Geometry: final body of the model. Coordinates: model frame, mm. A direction names the side the tool comes from. Give positions to 0.01 mm unless a question says otherwise; leave off trailing zeros. Loops run counter-clockwise (first coordinate to the right, second up) from the corner with the lowest first, then second, coordinate; pieces in that order, holes last. Notation, with made-up numbers: M -32.75,87 L -23.75,87 A34 cw -23.75,119 Z; hole C 58.5,-23 d1. An arc over 180 degrees is marked long. Put each result on its own line as item: value.
```python
from build123d import *

# Parameters (mm, degrees)
SKETCH1_W                       = 40.64
SKETCH1_H                       = 17.78
BOSS_EXTRUDE1_DEPTH             = 29.972
SKETCH2_W                       = 26.67
SKETCH2_H                       = 29.972
CUT_EXTRUDE1_DEPTH              = 12.7
SKETCH5_R                       = 8.001
CUT_EXTRUDE4_DEPTH              = 41.340446006
SKETCH6_R                       = 1.1303
CUT_EXTRUDE5_DEPTH              = 52.802457789
SKETCH7_W                       = 19.900329636
SKETCH7_H                       = 4.576555205
BOSS_EXTRUDE2_DEPTH             = 5.08
F_5_32_0_15625_DIAMETER_HOLE1_D = 3.96875
F_30_0_1285_DIAMETER_HOLE1_D    = 3.2639
SKETCH14_W                      = 1.1303
SKETCH14_H                      = 29.972
SKETCH16_W                      = 40.64
SKETCH16_H                      = 26.629644064
CUT_EXTRUDE6_DEPTH              = 41.347520619


with BuildPart() as part:
    # Sketch1 → Boss-Extrude1 (new body)
    with BuildSketch(Plane(origin=(0, 0, 0), x_dir=(1, 0, 0), z_dir=(0, 1, 0))):
        with Locations((0, 2.667)):
            Rectangle(SKETCH1_W, SKETCH1_H)
    extrude(amount=BOSS_EXTRUDE1_DEPTH)

    # Sketch2 → Cut-Extrude1 (cut)
    with BuildSketch(Plane.XY.offset(6.223)):
        with Locations((0, 14.986)):
            Rectangle(SKETCH2_W, SKETCH2_H)
    extrude(amount=-CUT_EXTRUDE1_DEPTH, mode=Mode.SUBTRACT)

    # Sketch5 → Cut-Extrude4 (cut, through all)
    with BuildSketch(Plane(origin=(0, 0, -11.557), x_dir=(-1, 0, 0), z_dir=(0, 0, -1))):
        with Locations((0, 15.875)):
            Circle(SKETCH5_R)
    extrude(amount=-CUT_EXTRUDE4_DEPTH, mode=Mode.SUBTRACT)

    # Sketch6 → Cut-Extrude5 (cut, through all)
    with BuildSketch(Plane.ZY.offset(20.32)):
        with Locations((-2.667, 15.24)):
            Circle(SKETCH6_R)
    extrude(amount=-CUT_EXTRUDE5_DEPTH, mode=Mode.SUBTRACT)

    # Sketch7 → Boss-Extrude2 (add)
    with BuildSketch(Plane.XY.offset(-6.477)):
        with Locations((0, 27.693243708)):
            Rectangle(SKETCH7_W, SKETCH7_H)
    extrude(amount=BOSS_EXTRUDE2_DEPTH)

    # 5/32 (0.15625) Diameter Hole1 (through all)
    with Locations(Plane(origin=(0, 0, -11.557), x_dir=(-1, 0, 0), z_dir=(0, 0, -1))):
        with Locations((-10.16, 21.717), (-10.16, 10.033), (10.16, 21.717), (10.16, 10.033)):
            Hole(F_5_32_0_15625_DIAMETER_HOLE1_D / 2)

    # #30 (0.1285) Diameter Hole1 (through all)
    with Locations(Plane(origin=(0, 29.972, 0), x_dir=(-1, 0, 0), z_dir=(0, 1, 0))):
        with Locations((16.8275, 3.048), (16.8275, -8.382), (-16.8275, -8.382), (-16.8275, 3.048)):
            Hole(F_30_0_1285_DIAMETER_HOLE1_D / 2)

    # Sketch14 → #4-40 Tapped Hole1 (revolve, cut)
    with BuildSketch(Plane(origin=(0, 29.972, -3.937), x_dir=(0, 0, 1), z_dir=(1, 0, 0))):
        with Locations((0.56515, 14.986)):
            Rectangle(SKETCH14_W, SKETCH14_H)
    revolve(axis=Axis((0, 36.322, -3.937), (0, -1, 0)), mode=Mode.SUBTRACT)

    # Sketch16 → Cut-Extrude6 (cut, through all)
    with BuildSketch(Plane(origin=(0, 0, -11.557), x_dir=(-1, 0, 0), z_dir=(0, 0, -1))):
        with Locations((0, 18.902822032)):
            Rectangle(SKETCH16_W, SKETCH16_H)
    extrude(amount=-CUT_EXTRUDE6_DEPTH, mode=Mode.SUBTRACT)


solid = part.part
```
Item 1: Line query: probe 1 along X at (y, z) = (0.6, 1) (3 decimals); probe 2 along X at (y, z) = (3.2, 4) (3 decimals); probe 3 along Z at (x, y) = (2, 2.1). Output: solid intervals per line, ascending. Write a range as [from, to].
Output values:
probe 1: [-20.32, -13.335], [13.335, 20.32]
probe 2: [-20.32, -18.153], [-15.502, -13.335], [13.335, 15.502], [18.153, 20.32]
probe 3: [-11.56, -6.48]
Item 2: Pin query (flat end, axial travel): pin 1 Ø1.7 at (x, y) = (-6, 3) entering from +Z. Return the tip coordinate at first contact, or that it passes through.
Output values:
pin 1: z = -6.48
Item 3: Section D-D on y = 3.8. Output: boundary loops of the cut face in (x, z) (1 decimal).
Output values:
outline: M -20.3,-11.6 L 20.3,-11.6 L 20.3,6.2 L 13.3,6.2 L 13.3,-6.5 L -13.3,-6.5 L -13.3,6.2 L -20.3,6.2 Z; hole C -16.8,-8.4 d3.3; hole C -16.8,3 d3.3; hole C 16.8,-8.4 d3.3; hole C 16.8,3 d3.3
Item 4: Section A-A on z = -1.5. Output: boundary loops of the cut face in (x, y) (3 decimals), then the cut area to 3 significant figures.
Output values:
outline: M -20.32,0 L -13.335,0 L -13.335,5.588 L -20.32,5.588 Z; M 13.335,0 L 20.32,0 L 20.32,5.588 L 13.335,5.588 Z
area: 78.1 mm²
Item 5: Section B-B on x = 16. Output: boundary loops of the cut face in (y, z).
Output values:
outline: M 0,-11.56 L 5.59,-11.56 L 5.59,-9.79 L 0,-9.79 Z; M 0,-6.98 L 5.59,-6.98 L 5.59,1.64 L 0,1.64 Z; M 0,4.45 L 5.59,4.45 L 5.59,6.22 L 0,6.22 Z
Item 6: Mould query, pull axis Z, two halves, no side actions, for faces 1 (the flat face through (17, 3, 6.223)), 2 (the flat face through (-13.335, 3, 0)), 3 (the cylindrical face through (-18.458, 2.755, 3.12)). Classes: pulls with the +Z half, pulls with the -Z half, needs draft (parallel to the pull), parting line crosses it, or undercut.
Output values:
face 1: pulls with the +Z half
face 2: needs draft
face 3: undercut
Item 7: Set-up query: faces 4 (the flat face through (0, 3, -6.477)), 5 (the flat face through (20.32, 3, -3)). Return all of +Z, -Z, +X, -X, +Y, -Y with unobstructed straight access to the full face (end or side cutting, diameter ignored); none if empty.
Output values:
face 4: +Z, +Y, -Y
face 5: +Z, -Z, +X, +Y, -Y
Item 8: Section C-C on z = -9. Output: boundary loops of the cut face in (x, y), then the cut area to 3 significant figures.
Output values:
outline: M -20.32,0 L -18.34,0 L -18.34,5.59 L -20.32,5.59 Z; M -15.32,0 L 15.32,0 L 15.32,5.59 L -15.32,5.59 Z; M 18.34,0 L 20.32,0 L 20.32,5.59 L 18.34,5.59 Z
area: 193 mm²
